CAD build for the part. Positions are in the model's coordinates, mm. A direction names the side the tool comes from. Coordinates: 2 decimals unless noted, no trailing zeros. Order: outer loops, then holes, each group sorted by start corner. A loop starts at its lowest first (then second) coordinate and runs counter-clockwise, first axis right, second up. Notation, with made-up numbers: (30, 63) - (76, 63) arc R19 cw to (76, 89) - close; hole circle Ø11 at (61.5, 64.25). An arc over 180 degrees is marked (long way). Return JSON: item names as keys, results as strings.
from build123d import *

# Parameters (mm, degrees)
F0_R     = 89
F0_R_2   = 3
F0_R_3   = 19
F1_DEPTH = 3
F2_R     = 39.5
F2_R_2   = 19
F3_DEPTH = 50


# Not quite as in the source:
# - a fillet or chamfer that OpenCascade refuses, or shapes differently, is made with other operations: its cross-section is extruded or revolved along the edge and cut away or added


with BuildPart() as f1:
    # F0 (on Top) → F1 (new body)
    with BuildSketch(Plane.XY):
        Circle(F0_R)
        with Locations((-57.735026919, -30)):
            Circle(F0_R_2, mode=Mode.SUBTRACT)
        with Locations((57.735026919, -30)):
            Circle(F0_R_2, mode=Mode.SUBTRACT)
        Circle(F0_R_3, mode=Mode.SUBTRACT)
        with Locations((0, 70)):
            Circle(F0_R_2, mode=Mode.SUBTRACT)
    extrude(amount=F1_DEPTH)

    # F2 (on face) → F3 (join)
    with BuildSketch(Plane.XY.offset(3)):
        Circle(F2_R)
        Circle(F2_R_2, mode=Mode.SUBTRACT)
    extrude(amount=F3_DEPTH)

    # F4: fillet of radius 5 on 3 edges, made by hand

    # F4_s1 → F4_t2 (revolve, cut)
    with BuildSketch(Plane.XZ.offset(30)):
        with BuildLine():
            ThreePointArc((60.735026919, 3), (62.5789898264, 0.8166998673), (65.3176026139, 0))
            Line((65.3176026139, 0), (60.735026919, 0))
            Line((60.735026919, 0), (60.735026919, 3))
        make_face()
    revolve(axis=Axis((57.735026919, -30, 0), (0, 0, 1)), mode=Mode.SUBTRACT)

    # F4_s3 → F4_t4 (revolve, cut)
    with BuildSketch(Plane.XZ.offset(-70)):
        with BuildLine():
            ThreePointArc((3, 3), (4.8439629074, 0.8166998673), (7.582575695, 0))
            Line((7.582575695, 0), (3, 0))
            Line((3, 0), (3, 3))
        make_face()
    revolve(axis=Axis((0, 70, 0), (0, 0, 1)), mode=Mode.SUBTRACT)

    # F4_s5 → F4_t6 (revolve, cut)
    with BuildSketch(Plane.XZ.offset(30)):
        with BuildLine():
            ThreePointArc((-54.735026919, 3), (-52.8910640115, 0.8166998673), (-50.152451224, 0))
            Line((-50.152451224, 0), (-54.735026919, 0))
            Line((-54.735026919, 0), (-54.735026919, 3))
        make_face()
    revolve(axis=Axis((-57.735026919, -30, 0), (0, 0, 1)), mode=Mode.SUBTRACT)


solid = f1.part
Item 1: Band-saw the part on D-D, the plane x = -36. List the corners of the cut face in (y, z), then the cut area to 3 significant figures.
Findings below:
{"outline": "(-81.39, 0) - (81.39, 0) - (81.39, 3) - (16.26, 3) - (16.26, 53) - (-16.26, 53) - (-16.26, 3) - (-81.39, 3) - close", "area": "2,110 mm²"}
Item 2: Drop flat-ended pins along their axis: P1, Ø4, axis at x = 12, y = 70, coming from the +Z side; P2, Ø3, axis at y = 17.5, z = 23, coming from the -X side; P3, Ø4, axis at y = -33.5, z = 15, coming from the -X side; P4, Ø2, axis at x = 58.5, y = -70, coming from the -Z side. Give the stop position or say it passes through.
Findings below:
{"P1": "stops at z = 3", "P2": "stops at x = -36.11", "P3": "stops at x = -23.83", "P4": "passes through"}
Item 3: Wall check: L1, parallel to Y at x = 0, z = 36; L2, parallel to Z at x = -46.5, y = 71; L3, parallel to X at y = -9.5, z = 35. Give the ranges that are in metal, low to high. Write a range as [from, to].
Findings below:
{"L1": "y = [-39.5, -19], [19, 39.5]", "L2": "z = [0, 3]", "L3": "x = [-38.34, -16.45], [16.45, 38.34]"}
Item 4: Band-saw the part on B-B, the plane y = 0. List the corners of the cut face in (x, z), then the cut area to 3 significant figures.
Findings below:
{"outline": "(-89, 0) - (-19, 0) - (-19, 53) - (-39.5, 53) - (-39.5, 3) - (-89, 3) - close; (19, 0) - (89, 0) - (89, 3) - (39.5, 3) - (39.5, 53) - (19, 53) - close", "area": "2,470 mm²"}
Item 5: Which spindle directions (+Z, -Z, +X, -X, +Y, -Y) get a long thin tool onto all of the face, cutting with end or side? Do faces 4 (the cylindrical face through (-29.11, 26.7, 27.65)), 5 (the flat face through (-1, 21, 0)). Say none if no direction does.
Findings below:
{"face 4": "+Z", "face 5": "-Z, +X, -X, +Y, -Y"}
Item 6: Band-saw the part on A-A, the plane x = 0. List the corners of the cut face in (y, z).
Findings below:
{"outline": "(-89, 0) - (-19, 0) - (-19, 53) - (-39.5, 53) - (-39.5, 3) - (-89, 3) - close; (19, 0) - (62.42, 0) arc R5 ccw to (67, 3) - (39.5, 3) - (39.5, 53) - (19, 53) - close; (73, 3) arc R5 ccw to (77.58, 0) - (89, 0) - (89, 3) - close"}
Item 7: Mould opens along Y. For faces 1 (the cylindrical face through (8.767, -16.856, 26.129)), 2 (the cylindrical face through (-65.597, 60.15, 1.479)), 3 (the flat face through (-9, -17, 53)) say: released by +Y, released by -Y, zero draft, split by the parting line, or undercut.
Findings below:
{"face 1": "undercut", "face 2": "split by the parting line", "face 3": "zero draft"}
Item 8: Band-saw the part on C-C, the plane z = 26. List the corners of the cut face in (x, y).
Findings below:
{"outline": "circle Ø79 at (0, 0); hole circle Ø38 at (0, 0)"}
